CAD build for the part. Positions are in the model's coordinates, mm. Give positions to 0.01 mm unless a question says otherwise; leave off trailing zeros. Answer as a JSON object with one key per item and string values.
```python
from build123d import *

# Parameters (mm, degrees)
F0_R     = 127
F0_R_2   = 11.1125
F0_R_3   = 57.15
F1_DEPTH = 30.226
F2_R     = 76.2
F2_R_2   = 57.15
F3_DEPTH = 1.905
F4_R     = 1.90499


# Not quite as in the source:
# - a fillet or chamfer is up to 0.001 mm smaller than in the source, because OpenCascade refuses the exact size


with BuildPart() as f1:
    # F0 (on Front) → F1 (new body)
    with BuildSketch(Plane.XZ):
        Circle(F0_R)
        with Locations((-38.2974271774, -92.4581680956)):
            Circle(F0_R_2, mode=Mode.SUBTRACT)
        with Locations((-92.4581680956, -38.2974271774)):
            Circle(F0_R_2, mode=Mode.SUBTRACT)
        with Locations((38.2974271774, -92.4581680956)):
            Circle(F0_R_2, mode=Mode.SUBTRACT)
        with Locations((92.4581680956, -38.2974271774)):
            Circle(F0_R_2, mode=Mode.SUBTRACT)
        with Locations((-92.4581680956, 38.2974271774)):
            Circle(F0_R_2, mode=Mode.SUBTRACT)
        with Locations((-38.2974271774, 92.4581680956)):
            Circle(F0_R_2, mode=Mode.SUBTRACT)
        Circle(F0_R_3, mode=Mode.SUBTRACT)
        with Locations((92.4581680956, 38.2974271774)):
            Circle(F0_R_2, mode=Mode.SUBTRACT)
        with Locations((38.2974271774, 92.4581680956)):
            Circle(F0_R_2, mode=Mode.SUBTRACT)
    extrude(amount=F1_DEPTH)

    # F2 (on face) → F3 (join)
    with BuildSketch(Plane.XZ.offset(30.226)):
        Circle(F2_R)
        Circle(F2_R_2, mode=Mode.SUBTRACT)
    extrude(amount=F3_DEPTH)

    # F4 (radius 1.905 in the source; OpenCascade refuses exactly that, so slightly less here)
    f4_edges = [f1.edges().sort_by_distance(p)[0] for p in [
        (-127, 0, 0),
        (-127, -30.226, 0),
        (-76.2, -32.131, 0),
    ]]
    fillet(f4_edges, radius=F4_R)


solid = f1.part
```
1) Slice it at C-C (y = -11). State how many separate pieces and enclosed holes the cut face has, then the cut area to 3 significant figures.
Model answer:
{"separate pieces": "1", "enclosed holes": "9", "area": "37,300 mm2"}
2) Mould opens along X. For faces 1 (the cylindrical face through (-27.53, -14.93, -123.98)), 2 (the flat face through (-57, -30.226, -54)), 3 (the cylindrical face through (-57.095, -15.841, 2.513)) say: released by +X, released by -X, zero draft, split by the parting line, or undercut.
Model answer:
{"face 1": "split by the parting line", "face 2": "zero draft", "face 3": "undercut"}
3) Wall check: probe 1 along X at (y, z) = (-28, -33.5); probe 2 along Z at (x, y) = (82.5, -27.5); probe 3 along Y at (x, z) = (32.5, -72). Give the ranges that are in metal, low to high.
Model answer:
{"probe 1": "x = -122.5 to -102.48, -82.43 to -46.3, 46.3 to 82.43, 102.48 to 122.5", "probe 2": "z = -96.55 to -43.23, -33.37 to 33.37, 43.23 to 96.55", "probe 3": "y = -30.23 to 0"}
4) Pin check, flat tips, straight feed: pin 1 (1.5 mm diameter, centred on y = -5.5, z = 28, fed in from +X); pin 2 (6 mm diameter, centred on y = -13, z = -8, fed in from -X); pin 3 (18 mm diameter, centred on x = -92.46, z = -38.3, fed in from +Y); pin 4 (2 mm diameter, centred on x = 58, y = -3.5, fed in from -Z). Stop position of each tip, or through.
Model answer:
{"pin 1": "stops at x = 124.04", "pin 2": "stops at x = -126.9", "pin 3": "passes through", "pin 4": "stops at z = -113.49"}
